```python
from build123d import *

# Parameters (mm, degrees)
SKETCH2_R           = 25.4
BOSS_EXTRUDE2_DEPTH = 12.7
CUT_EXTRUDE2_DEPTH  = 17.272


with BuildPart() as part:
    # Sketch2 → Boss-Extrude2 (new body)
    with BuildSketch(Plane.XY):
        Circle(SKETCH2_R)
    extrude(amount=BOSS_EXTRUDE2_DEPTH)

    # Cut-Sweep2: sweep along a curve in space
    with BuildLine() as cut_sweep2_path:
        ThreePointArc((25.4, 0, 12.7), (17.960512242, 17.960512242, 12.7), (0, 25.4, 12.7))
        ThreePointArc((0, 25.4, 12.7), (-17.960512242, 17.960512242, 12.7), (-25.4, 0, 12.7))
        ThreePointArc((-25.4, 0, 12.7), (-17.960512242, -17.960512242, 12.7), (0, -25.4, 12.7))
        ThreePointArc((0, -25.4, 12.7), (17.960512242, -17.960512242, 12.7), (25.4, 0, 12.7))
    # Sketch3 → Cut-Sweep2 (sweep, cut)
    with BuildSketch(Plane(origin=(0, 0, 0), x_dir=(0, 0, -1), z_dir=(1, 0, 0))):
        with BuildLine():
            Line((-12.065, 25.4), (-0.635, 25.4))
            ThreePointArc((-0.635, 25.4), (-6.35, 19.685), (-12.065, 25.4))
        make_face()
    sweep(path=cut_sweep2_path.line, mode=Mode.SUBTRACT)

    # Sketch22 → Cut-Extrude2 (cut)
    with BuildSketch(Plane.XY):
        Polygon((7.332348419, 0), (3.666174209, 6.35), (-3.666174209, 6.35), (-7.332348419, 0), (-3.666174209, -6.35), (3.666174209, -6.35), align=None)
    extrude(amount=CUT_EXTRUDE2_DEPTH, mode=Mode.SUBTRACT)


solid = part.part
```
For this review, take the finished solid that the model builds, in its own axes (mm). A direction names the side the tool comes from. Coordinates: 2 decimals unless noted, no trailing zeros. Order: outer loops, then holes, each group sorted by start corner. A loop starts at its lowest first (then second) coordinate and runs counter-clockwise, first axis right, second up. Notation, with made-up numbers: (16.25, -14.75) - (52.25, -14.75) arc R20 ccw to (52.25, 15.25) - close; hole circle Ø1 at (-2.75, 5). An arc over 180 degrees is marked (long way). Answer as a JSON object with one key per item and string values. Group by question number.
1. For probe 1 along Z at (x, y) = (20, 12.5); probe 2 along X at (y, z) = (2, 10.25); probe 3 along X at (y, z) = (-2, 0.5), list the stretches that pass through material, from the lowest coordinate up.
2. Clearance check with flat-ended pins moving along their axes: P1, Ø2, axis at x = 0, z = 5, coming from the +Y side; P2, Ø5, axis at x = -1, z = 4, coming from the -Y side; P3, Ø3, axis at y = -9, z = 9.5, coming from the -X side. State where each tip first meets the part, or that it passes through.
3. For faces 5 (the flat face through (5, -5, 0)), 6 (the flat face through (-5.474, 3.219, 6.261)), list the 3-axis set-ups (+Z, -Z, +X, -X, +Y, -Y) from which the entire face can be reached by the end or side of a thin tool; tool diameter is ignored.
4. We need section B-B on z = 6.5. State the section outline as (x, y) points.
5. We need section A-A on z = 9.25. State the section outline as (x, y) points.
6. The part is to be moulded in two halves that separate along Y. For faces 1 (the flat face through (5, -5, 12.7)), 2 (the cylindrical face through (-5.506, -24.796, 12.378)), 3 (the flat face through (-5.525, -3.131, 6.261)), 4 (the flat face through (5.525, 3.131, 6.261)), say which applies: pulls with the +Y half, pulls with the -Y half, needs draft (parallel to the pull), parting line crosses it, or undercut.
Final values:
{
 "1": {"probe 1": "0 to 0.93, 11.77 to 12.7", "probe 2": "-21.13 to -6.18, 6.18 to 21.13", "probe 3": "-25.32 to -6.18, 6.18 to 25.32"},
 "2": {"P1": "y = 20.19", "P2": "y = -22.36", "P3": "x = -20.25"},
 "3": {"face 5": "-Z, +X, -X, +Y, -Y", "face 6": "+Z, -Z"},
 "4": {"outline": "circle Ø39.37 at (0, 0); hole (-7.33, 0) - (-3.67, -6.35) - (3.67, -6.35) - (7.33, 0) - (3.67, 6.35) - (-3.67, 6.35) - close"},
 "5": {"outline": "circle Ø40.95 at (0, 0); hole (-7.33, 0) - (-3.67, -6.35) - (3.67, -6.35) - (7.33, 0) - (3.67, 6.35) - (-3.67, 6.35) - close"},
 "6": {"face 1": "needs draft", "face 2": "parting line crosses it", "face 3": "undercut", "face 4": "undercut"}
}
